Could you check a few things on this model? Use its own coordinates, in mm. A direction names the side the tool comes from. Give positions to 0.01 mm unless a question says otherwise; leave off trailing zeros. Write each loop counter-clockwise with the first axis right and the second up, starting at its lowest first coordinate (ties: lowest second). Pieces come first, ordered by that corner, then holes. Notation, with made-up numbers: (89, 73) - (144, 73) arc R22 cw to (144, 109) - close; hole circle Ø8 at (37, 85). An arc over 180 degrees is marked (long way). Answer as CSV lines item,"result". Start each with the question number.
Q1. Imagine slicing it at C-C on z = 0.8. State how many separate pieces and enclosed holes the cut face has, and give its area (3 significant figures).
Q2. Imagine slicing it at D-D on x = -29. List the corners of the cut face in (y, z) for me (1 decimal), and give its area (3 significant figures).
Q3. Imagine slicing it at A-A on y = 72.39. List the corners of the cut face in (x, z) for me (1 decimal).
Q4. If I drill on line 1 along Y through (x, z) = (-34, 0.8) (1 decimal); line 2 along Y through (x, z) = (-29, 2.85) (1 decimal); line 3 along Y through (x, z) = (-32.5, 1.65) (1 decimal), over which ranges is the centre line in solid material (lowest first)?
Q5. Imagine slicing it at B-B on x = -22. List the corners of the cut face in (y, z) for me (1 decimal), and give its area (3 significant figures).
Q6. We'd pull the mould along X, two halves only. Please class faces 1 (the face through (-29, 90, 0)), 2 (the face through (-54.928, 85, 2)), 3 (the face through (-26.74, 125.055, 2.348)): pulls with the +X half, pulls with the -X half, needs draft (parallel to the pull), parting line crosses it, or undercut.
Q7. Will these pins go through, and if not, where does the flat tip stop? pin 1 Ø7 at (x, y) = (-28.448, 126.365) entering from -Z; pin 2 Ø1 at (x, z) = (-52.5, 2.5) entering from +Y; pin 3 Ø1.7 at (y, z) = (132, 3.5) entering from -X.
Q8. On a 3-axis mill with a long thin cutter (end or side, diameter ignored), from which of +Z, -Z, +X, -X, +Y, -Y can I reach the whole of each face in a straight line? I mean faces 4 (the face through (-20.92, 110.83, 2.35)), 5 (the face through (-45.212, 132, 2)). Say none if no direction works.
```python
from build123d import *

# Parameters (mm, degrees)
BOSS_EXTRUDE1_DEPTH         = 4.7625
F_6_CLEARANCE_HOLE1_D       = 4.3053
F_3_4_0_75_DIAMETER_HOLE1_D = 19.05


with BuildPart() as part:
    # Sketch1 → Boss-Extrude1 (new body)
    with BuildSketch(Plane.XY):
        with BuildLine():
            Line((-50.8, 124.587), (-54.1655, 124.587))
            ThreePointArc((-54.1655, 124.587), (-54.704315367, 124.363815367), (-54.9275, 123.825))
            Line((-54.9275, 123.825), (-54.9275, 44.577))
            ThreePointArc((-54.9275, 44.577), (-54.704315367, 44.038184633), (-54.1655, 43.815))
            Line((-54.1655, 43.815), (-3.302, 43.815))
            ThreePointArc((-3.302, 43.815), (-2.763184633, 44.038184633), (-2.54, 44.577))
            Line((-2.54, 44.577), (-2.54, 133.5405))
            ThreePointArc((-2.54, 133.5405), (-2.763184633, 134.079315367), (-3.302, 134.3025))
            Line((-3.302, 134.3025), (-44.45, 134.3025))
            ThreePointArc((-44.45, 134.3025), (-44.988815367, 134.079315367), (-45.212, 133.5405))
            Line((-45.212, 133.5405), (-45.212, 130.175))
            ThreePointArc((-45.212, 130.175), (-46.848687307, 126.223687307), (-50.8, 124.587))
        make_face()
    extrude(amount=BOSS_EXTRUDE1_DEPTH)

    # #6 Clearance Hole1 (through all)
    with Locations(Plane.XY.offset(4.7625)):
        with Locations((-28.448, 126.365), (-28.448, 51.7525)):
            Hole(F_6_CLEARANCE_HOLE1_D / 2)

    # 3/4 (0.75) Diameter Hole1 (through all)
    with Locations(Plane.XY.offset(4.7625)):
        with Locations((-27.94, 72.39), (-27.94, 104.394)):
            Hole(F_3_4_0_75_DIAMETER_HOLE1_D / 2)


solid = part.part
```
Conclusion:
1,separate pieces,"1"
1,enclosed holes,"4"
1,area,"4,050 mm^2"
2,outline,"(43.8, 0) - (49.7, 0) - (49.7, 4.8) - (43.8, 4.8) - close; (53.8, 0) - (62.9, 0) - (62.9, 4.8) - (53.8, 4.8) - close; (81.9, 0) - (94.9, 0) - (94.9, 4.8) - (81.9, 4.8) - close; (113.9, 0) - (124.3, 0) - (124.3, 4.8) - (113.9, 4.8) - close; (128.4, 0) - (134.3, 0) - (134.3, 4.8) - (128.4, 4.8) - close"
2,area,"211 mm^2"
3,outline,"(-54.9, 0) - (-37.5, 0) - (-37.5, 4.8) - (-54.9, 4.8) - close; (-18.4, 0) - (-2.5, 0) - (-2.5, 4.8) - (-18.4, 4.8) - close"
4,line 1,"43.8 to 65, 79.7 to 97, 111.7 to 134.3"
4,line 2,"43.8 to 49.7, 53.8 to 62.9, 81.9 to 94.9, 113.9 to 124.3, 128.4 to 134.3"
4,line 3,"43.8 to 64, 80.8 to 96, 112.8 to 134.3"
5,outline,"(43.8, 0) - (64.9, 0) - (64.9, 4.8) - (43.8, 4.8) - close; (79.8, 0) - (96.9, 0) - (96.9, 4.8) - (79.8, 4.8) - close; (111.8, 0) - (134.3, 0) - (134.3, 4.8) - (111.8, 4.8) - close"
5,area,"289 mm^2"
6,face 1,"needs draft"
6,face 2,"pulls with the -X half"
6,face 3,"undercut"
7,pin 1,"z = 0"
7,pin 2,"y = 124.59"
7,pin 3,"x = -45.21"
8,face 4,"+Z, -Z"
8,face 5,"+Z, -Z, -X, +Y"
